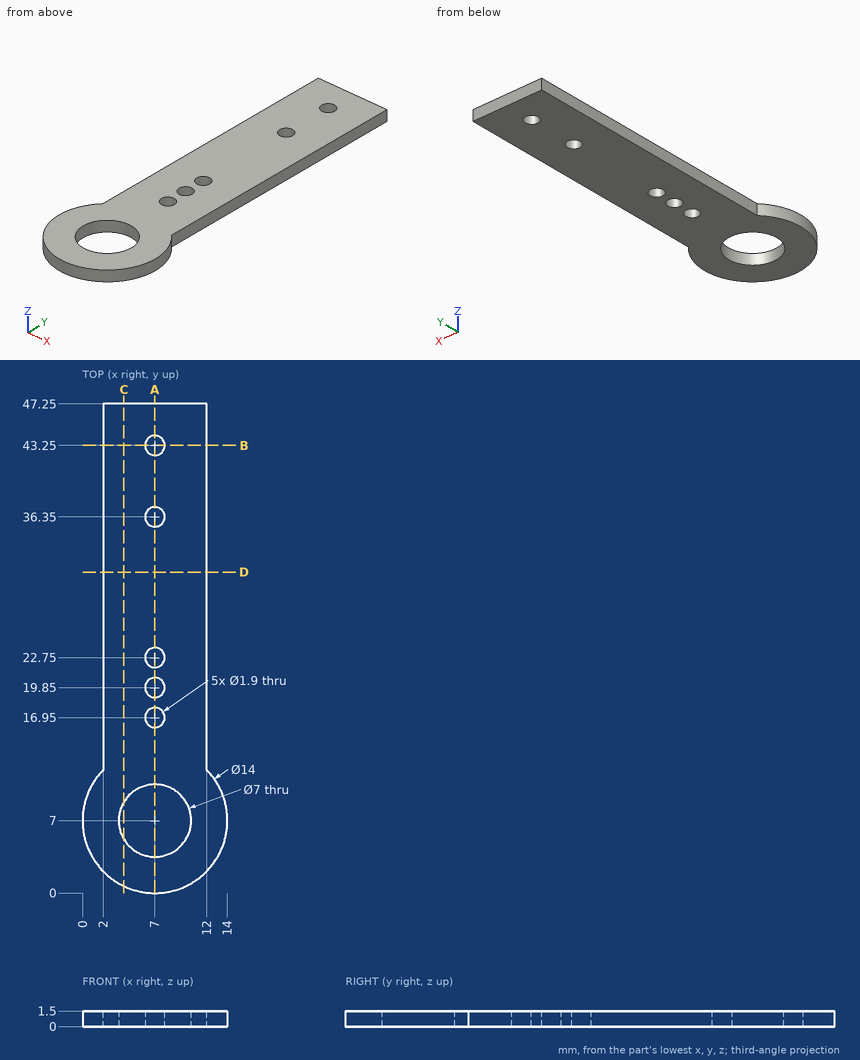
The drawing under review shows one solid part. Ordinate dimensions are in mm from its lowest x, y, z. Coordinates: 2 decimals unless noted, no trailing zeros. Write each loop counter-clockwise with the first axis right and the second up, starting at its lowest first coordinate (ties: lowest second). Pieces come first, ordered by that corner, then holes. Notation, with made-up numbers: (18.25, 15.5) - (50.25, 15.5) arc R24 ccw to (50.25, 44.5) - close; hole circle Ø5 at (33.5, -32.5). An arc over 180 degrees is marked (long way). Answer in a Markdown table with one row per item. Add a question column.
Q1. We need section D-D, the plane y = 31. State the section outline as (x, z) points.
Q2. We need section A-A, the plane x = 7. State the section outline as (y, z) points, and give its area (3 significant figures).
Q3. For probe 1 along X at (y, z) = (43.25, 1.15); probe 2 along Y at (x, z) = (9.75, 1.2); probe 3 along X at (y, z) = (21.5, 0.9), list the stretches that pass through material, from the lowest coordinate up.
Q4. We need section C-C, the plane x = 4. State the section outline as (y, z) points, and give its area (3 significant figures).
Q5. We need section B-B, the plane y = 43.25. State the section outline as (x, z) points, and give its area (4 significant figures).
Q6. For P1, Ø0.8, axis at y = 21.5, z = 1, coming from the +X side, flat-tipped, find the tip position at first contact; note if it passes through.
Answer list:
| question | item | result |
|---|---|---|
| 1 | outline | (2, 0) - (12, 0) - (12, 1.5) - (2, 1.5) - close |
| 2 | outline | (0, 0) - (3.5, 0) - (3.5, 1.5) - (0, 1.5) - close; (10.5, 0) - (16, 0) - (16, 1.5) - (10.5, 1.5) - close; (17.9, 0) - (18.9, 0) - (18.9, 1.5) - (17.9, 1.5) - close; (20.8, 0) - (21.8, 0) - (21.8, 1.5) - (20.8, 1.5) - close; (23.7, 0) - (35.4, 0) - (35.4, 1.5) - (23.7, 1.5) - close; (37.3, 0) - (42.3, 0) - (42.3, 1.5) - (37.3, 1.5) - close; (44.2, 0) - (47.25, 0) - (47.25, 1.5) - (44.2, 1.5) - close |
| 2 | area | 46.1 mm2 |
| 3 | probe 1 | x = 2 to 6.05, 7.95 to 12 |
| 3 | probe 2 | y = 0.56 to 4.83, 9.17 to 47.25 |
| 3 | probe 3 | x = 2 to 12 |
| 4 | outline | (0.68, 0) - (5.2, 0) - (5.2, 1.5) - (0.68, 1.5) - close; (8.8, 0) - (47.25, 0) - (47.25, 1.5) - (8.8, 1.5) - close |
| 4 | area | 64.5 mm2 |
| 5 | outline | (2, 0) - (6.05, 0) - (6.05, 1.5) - (2, 1.5) - close; (7.95, 0) - (12, 0) - (12, 1.5) - (7.95, 1.5) - close |
| 5 | area | 12.15 mm2 |
| 6 | P1 | stops at x = 12 |
